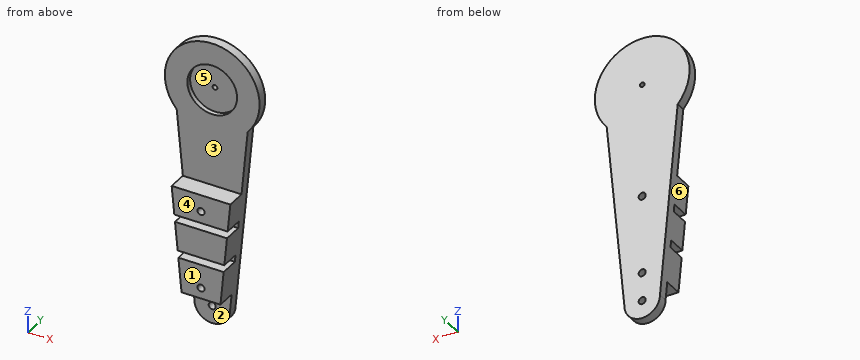
from build123d import *

# Parameters (mm, degrees)
SKETCH2_R           = 1
CUT_EXTRUDE1_DEPTH  = 10
BOSS_EXTRUDE1_DEPTH = 4
BOSS_EXTRUDE2_DEPTH = 8
SKETCH5_R           = 1.5
CUT_EXTRUDE2_DEPTH  = 12
SKETCH6_R           = 7.5
BOSS_EXTRUDE3_DEPTH = 12
CUT_EXTRUDE3_DEPTH  = 8
SKETCH8_R           = 1.5
CUT_EXTRUDE4_DEPTH  = 4


with BuildPart() as part:
    # Sketch1 → Revolve1 (revolve)
    with BuildSketch(Plane.XY):
        Polygon((0, -2), (10.5, -2), (10.5, -4), (20, -4), (20, 0), (0, 0), align=None)
    revolve(axis=Axis((0, 0, 0), (0, -1, 0)))

    # Sketch2 → Cut-Extrude1 (cut)
    with BuildSketch(Plane(origin=(0, 0, 0), x_dir=(1, 0, 0), z_dir=(0, 1, 0))):
        Circle(SKETCH2_R)
    extrude(amount=-CUT_EXTRUDE1_DEPTH, mode=Mode.SUBTRACT)

    # Sketch3 → Boss-Extrude1 (add)
    with BuildSketch(Plane(origin=(0, 0, 0), x_dir=(1, 0, 0), z_dir=(0, 1, 0))):
        Polygon((-7.5, 93), (-15, 13), (15, 13), (7.5, 93), align=None)
    extrude(amount=-BOSS_EXTRUDE1_DEPTH)

    # Sketch4 → Boss-Extrude2 (add)
    with BuildSketch(Plane.XZ.offset(4)):
        Polygon((-12.375, -41), (12.375, -41), (11.25, -53), (-11.25, -53), align=None)
        Polygon((-10.96875, -56), (10.96875, -56), (9.84375, -68), (-9.84375, -68), align=None)
        Polygon((-9.5625, -71), (9.5625, -71), (7.5, -93), (-7.5, -93), align=None)
    extrude(amount=BOSS_EXTRUDE2_DEPTH)

    # Sketch5 → Cut-Extrude2 (cut)
    with BuildSketch(Plane(origin=(0, 0, 0), x_dir=(1, 0, 0), z_dir=(0, 1, 0))):
        with Locations((0, 48)):
            Circle(SKETCH5_R)
        with Locations((0, 81)):
            Circle(SKETCH5_R)
    extrude(amount=-CUT_EXTRUDE2_DEPTH, mode=Mode.SUBTRACT)

    # Sketch6 → Boss-Extrude3 (add)
    with BuildSketch(Plane.XZ.offset(12)):
        with Locations((0, -93)):
            Circle(SKETCH6_R)
    extrude(amount=-BOSS_EXTRUDE3_DEPTH)

    # Sketch7 → Cut-Extrude3 (cut)
    with BuildSketch(Plane.XZ.offset(12)):
        with BuildLine():
            Line((-8.203125, -85.5), (8.203125, -85.5))
            Line((8.203125, -85.5), (7.5, -93))
            ThreePointArc((7.5, -93), (0, -100.5), (-7.5, -93))
            Line((-7.5, -93), (-8.203125, -85.5))
        make_face()
    extrude(amount=-CUT_EXTRUDE3_DEPTH, mode=Mode.SUBTRACT)

    # Sketch8 → Cut-Extrude4 (cut)
    with BuildSketch(Plane(origin=(0, 0, 0), x_dir=(1, 0, 0), z_dir=(0, 1, 0))):
        with Locations((0, 93)):
            Circle(SKETCH8_R)
    extrude(amount=-CUT_EXTRUDE4_DEPTH, mode=Mode.SUBTRACT)


solid = part.part
Part model, mm, in its own coordinate system. Face numbers are marked on the shaded views. A direction names the side the tool comes from. Round coordinates to 2 decimals unless told otherwise and drop trailing zeros. Order: outer loops, then holes, each group sorted by start corner. A loop starts at its lowest first (then second) coordinate and runs counter-clockwise, first axis right, second up. Notation, with made-up numbers: (43, 60) -> (92, 60) arc R25 cw to (92, 88) -> close; hole circle Ø3 at (60.25, 4.5). An arc over 180 degrees is marked (long way). Put each result on its own line as item: value.
Q1. Band-saw the part on D-D (z = 3.5). Give the cut face in (x, y), and give its area (3 significant figures).
From the geometry:
outline: (-19.69, -4) -> (-9.9, -4) -> (-9.9, -2) -> (9.9, -2) -> (9.9, -4) -> (19.69, -4) -> (19.69, 0) -> (-19.69, 0) -> close
area: 118 mm2
Q2. Tool access for the marked faces 1, 2 and 3: list every direction of +Z, -Z, +X, -X, +Y, -Y with a clear straight run to the whole face (end or side of a thin tool).
From the geometry:
face 1: +Z, -Z, +X, -X, -Y
face 2: -Z, +X, -X, -Y
face 3: +Z, +X, -X, -Y
Q3. Pull direction Z, two halves, no side cores. Call the marked faces 4, 5 and 6: pulls with the +Z half, pulls with the -Z half, needs draft (parallel to the pull), parting line crosses it, or undercut.
From the geometry:
face 4: needs draft
face 5: undercut
face 6: pulls with the -Z half
Q4. Band-saw the part on B-B (z = -81). Give the cut face in (x, y) (3 decimals).
From the geometry:
outline: (-8.625, -12) -> (-1.5, -12) -> (-1.5, 0) -> (-8.625, 0) -> close; (1.5, -12) -> (8.625, -12) -> (8.625, 0) -> (1.5, 0) -> close
Q5. Band-saw the part on A-A (y = -6.25). State how many separate pieces and enclosed holes the cut face has, and give its area (3 significant figures).
From the geometry:
separate pieces: 3
enclosed holes: 2
area: 777 mm2
Q6. Band-saw the part on C-C (x = -4). Give the cut face in (y, z), and give its area (3 significant figures).
From the geometry:
outline: (-12, -85.5) -> (-4, -85.5) -> (-4, -99.34) -> (0, -99.34) -> (0, 19.6) -> (-4, 19.6) -> (-4, 9.71) -> (-2, 9.71) -> (-2, -9.71) -> (-4, -9.71) -> (-4, -41) -> (-12, -41) -> (-12, -53) -> (-4, -53) -> (-4, -56) -> (-12, -56) -> (-12, -68) -> (-4, -68) -> (-4, -71) -> (-12, -71) -> close
area: 745 mm2
Q7. Pin check, flat tips, straight feed: pin 1 Ø1 at (x, y) = (5.5, -6) entering from +Z; pin 2 Ø10.5 at (x, z) = (-0.5, 0.5) entering from -Y; pin 3 Ø4 at (x, y) = (1, -7) entering from -Z; pin 4 Ø1.8 at (x, z) = (0, 0) entering from +Y. Stop position of each tip, or through.
From the geometry:
pin 1: stops at z = -41
pin 2: stops at y = -2
pin 3: stops at z = -85.5
pin 4: passes through
Q8. Wall check: line 1 (Z direction, x = 0, y = -6.75); line 2 (Z direction, x = 6, y = -5.25); line 3 (X direction, y = -1.5, z = 0). Give the ranges that are in metal, low to high. Write a range as [from, to].
From the geometry:
line 1: z = [-85.5, -82.5], [-79.5, -71], [-68, -56], [-53, -49.5], [-46.5, -41]
line 2: z = [-85.5, -71], [-68, -56], [-53, -41]
line 3: x = [-20, -1], [1, 20]
